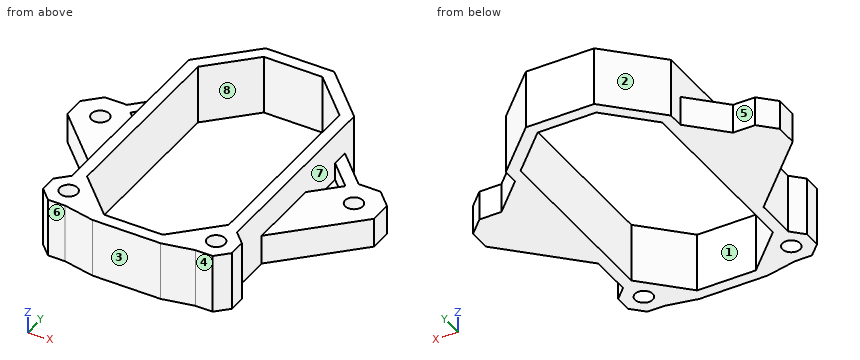
```python
from build123d import *

# Parameters (mm, degrees)
SKETCH2_R           = 1.5
BOSS_EXTRUDE1_DEPTH = 2
SKETCH5_R           = 1.5
BOSS_EXTRUDE4_DEPTH = 3
SKETCH6_R           = 1.5
BOSS_EXTRUDE5_DEPTH = 5


with BuildPart() as part:
    # Sketch2 → Boss-Extrude1 (new body)
    with BuildSketch(Plane.XY):
        Polygon((-26, -1.863961031), (-23.363961031, -4.5), (-14, -13.863961031), (-14, -20.798989873), (-14, -20.970562748), (-16, -22.970562748), (-16, -25.870057685), (-13.949747468, -27.920310217), (-11.050252532, -27.920310217), (-5.798989873, -29), (5.798989873, -29), (11.050252532, -27.920310217), (13.949747468, -27.920310217), (16, -25.870057685), (16, -22.970562748), (14, -20.970562748), (14, -20.798989873), (14, -13.863961031), (23.363961031, -4.5), (26, -1.863961031), (26, 1.863961031), (23.363961031, 4.5), (19.636038969, 4.5), (14, 10.136038969), (14, 12.798989873), (5.798989873, 21), (-5.798989873, 21), (-14, 12.798989873), (-14, 10.136038969), (-19.636038969, 4.5), (-23.363961031, 4.5), (-26, 1.863961031), align=None)
        with Locations((-12.5, -24.420310217)):
            Circle(SKETCH2_R, mode=Mode.SUBTRACT)
        with Locations(Location((12.5, -24.420310217, 0), (0, 0, 180))):
            Circle(SKETCH2_R, mode=Mode.SUBTRACT)
        Polygon((4.970562748, 19), (-4.970562748, 19), (-12, 11.970562748), (-12, 0), (-12, -19.970562748), (-4.970562748, -27), (4.970562748, -27), (12, -19.970562748), (12, 0), (12, 11.970562748), align=None, mode=Mode.SUBTRACT)
    extrude(amount=BOSS_EXTRUDE1_DEPTH)

    # Sketch5 → Boss-Extrude4 (add)
    with BuildSketch(Plane.XY.offset(2)):
        Polygon((-5.798989873, 21), (-14, 12.798989873), (-14, 10.136038969), (-19.636038969, 4.5), (-23.363961031, 4.5), (-26, 1.863961031), (-26, -1.863961031), (-23.363961031, -4.5), (-14, -13.863961031), (-14, -20.798989873), (-14, -20.970562748), (-16, -22.970562748), (-16, -25.870057685), (-13.949747468, -27.920310217), (-11.050252532, -27.920310217), (-5.798989873, -29), (5.798989873, -29), (11.050252532, -27.920310217), (13.949747468, -27.920310217), (16, -25.870057685), (16, -22.970562748), (14, -20.970562748), (14, -20.798989873), (14, -13.863961031), (23.363961031, -4.5), (26, -1.863961031), (26, 1.863961031), (23.363961031, 4.5), (19.636038969, 4.5), (14, 10.136038969), (14, 12.798989873), (5.798989873, 21), align=None)
        with Locations((-21.5, 0)):
            Circle(SKETCH5_R, mode=Mode.SUBTRACT)
        with Locations(Location((21.5, 0, 0), (0, 0, 180))):
            Circle(SKETCH5_R, mode=Mode.SUBTRACT)
        with Locations((-12.5, -24.420310217)):
            Circle(SKETCH5_R, mode=Mode.SUBTRACT)
        with Locations(Location((12.5, -24.420310217, 0), (0, 0, 180))):
            Circle(SKETCH5_R, mode=Mode.SUBTRACT)
        Polygon((-18.221825407, 3.085786438), (-14, 7.307611845), (-14, 0), (-14, -1.136038969), (-17, 1.863961031), align=None, mode=Mode.SUBTRACT)
        Polygon((4.970562748, -27), (-4.970562748, -27), (-12, -19.970562748), (-12, 0), (-12, 11.970562748), (-4.970562748, 19), (4.970562748, 19), (12, 11.970562748), (12, 0), (12, -19.970562748), align=None, mode=Mode.SUBTRACT)
        Polygon((14, -1.136038969), (14, 0), (14, 7.307611845), (18.221825407, 3.085786438), (17, 1.863961031), align=None, mode=Mode.SUBTRACT)
    extrude(amount=BOSS_EXTRUDE4_DEPTH)

    # Sketch6 → Boss-Extrude5 (add)
    with BuildSketch(Plane.XY.offset(5)):
        Polygon((5.798989873, -29), (-5.798989873, -29), (-11.050252532, -27.920310217), (-13.949747468, -27.920310217), (-16, -25.870057685), (-16, -22.970562748), (-14, -20.970562748), (-14, -20.798989873), (-14, 0), (-14, 12.798989873), (-5.798989873, 21), (5.798989873, 21), (14, 12.798989873), (14, 0), (14, -20.798989873), (14, -20.970562748), (16, -22.970562748), (16, -25.870057685), (13.949747468, -27.920310217), (11.050252532, -27.920310217), align=None)
        with Locations((-12.5, -24.420310217)):
            Circle(SKETCH6_R, mode=Mode.SUBTRACT)
        with Locations(Location((12.5, -24.420310217, 0), (0, 0, 180))):
            Circle(SKETCH6_R, mode=Mode.SUBTRACT)
        Polygon((4.970562748, 19), (-4.970562748, 19), (-12, 11.970562748), (-12, 0), (-12, -19.970562748), (-4.970562748, -27), (4.970562748, -27), (12, -19.970562748), (12, 0), (12, 11.970562748), align=None, mode=Mode.SUBTRACT)
    extrude(amount=BOSS_EXTRUDE5_DEPTH)


solid = part.part
```
The listing builds one solid part. Answer for the finished solid, in the listing's coordinates (mm). Face numbers are marked on the shaded views. A direction names the side the tool comes from. Coordinates: 2 decimals unless noted, no trailing zeros. Loops run counter-clockwise (first coordinate to the right, second up) from the corner with the lowest first, then second, coordinate; pieces in that order, holes last. Notation, with made-up numbers: (50.5, 48) -> (79.5, 48) arc R23 ccw to (79.5, 65) -> close; hole circle Ø3 at (28, 55.25). An arc over 180 degrees is marked (long way). Use one line per item in the form item = value. Start each with the question number.
Item 1: The part is cut by section A-A on x = 1. Determine the outline of the cut face in (y, z), then the cut area to 3 significant figures.
Item 2: Flat-ended cylindrical pins translate along their axes: pin 1 Ø2.5 at (x, y) = (-21.5, -0.5) entering from +Z; pin 2 Ø6 at (y, z) = (16, 8.5) entering from +X; pin 3 Ø2.5 at (y, z) = (-24.5, 6.5) entering from -X. Find the tip coordinate at first contact, or state that the pin passes through.
Item 3: The part is cut by section B-B on y = 13.5. Determine the outline of the cut face in (x, z).
Item 4: The mould has two halves that part along X. Classify the marked faces 1, 2 and 3: released by +X, released by -X, zero draft, split by the parting line, or undercut.
Item 5: The part is cut by section C-C on z = 6.5. Determine the outline of the cut face in (x, y).
Item 6: The part is cut by section D-D on y = -3.5. Determine the outline of the cut face in (x, z).
Item 7: Consider L1, parallel to X at y = 6.5, z = 6.25; L2, parallel to Y at x = 4, z = 3.5; L3, parallel to X at y = 17, z = 8. Determine where each line is inside the solid, lowest interval first. Write a range as [from, to].
Item 8: A tool of negligible diameter and unlimited length cuts with its end or side. For the marked faces 4, 5, 6, 7 and 8, from which of +Z, -Z, +X, -X, +Y, -Y can it reach the whole face along a straight path? Write none if from no direction.
Answer key:
q1.outline = (-29, 0) -> (-27, 0) -> (-27, 10) -> (-29, 10) -> close; (19, 0) -> (21, 0) -> (21, 10) -> (19, 10) -> close
q1.area = 40.0 mm2
q2.pin_1 = 5
q2.pin_2 = 13.8
q2.pin_3 = -16
q3.outline = (-13.3, 0) -> (-10.47, 0) -> (-10.47, 10) -> (-13.3, 10) -> close; (10.47, 0) -> (13.3, 0) -> (13.3, 10) -> (10.47, 10) -> close
q4.face_1 = undercut
q4.face_2 = released by -X
q4.face_3 = zero draft
q5.outline = (-16, -25.87) -> (-13.95, -27.92) -> (-11.05, -27.92) -> (-5.8, -29) -> (5.8, -29) -> (11.05, -27.92) -> (13.95, -27.92) -> (16, -25.87) -> (16, -22.97) -> (14, -20.97) -> (14, 12.8) -> (5.8, 21) -> (-5.8, 21) -> (-14, 12.8) -> (-14, -20.97) -> (-16, -22.97) -> close; hole circle Ø3 at (-12.5, -24.42); hole (-12, -19.97) -> (-4.97, -27) -> (4.97, -27) -> (12, -19.97) -> (12, 11.97) -> (4.97, 19) -> (-4.97, 19) -> (-12, 11.97) -> close; hole circle Ø3 at (12.5, -24.42)
q6.outline = (-24.36, 0) -> (-12, 0) -> (-12, 10) -> (-14, 10) -> (-14, 5) -> (-24.36, 5) -> close; (12, 0) -> (24.36, 0) -> (24.36, 5) -> (14, 5) -> (14, 10) -> (12, 10) -> close
q7.L1 = [-14, -12], [12, 14]
q7.L2 = [-29, -27], [19, 21]
q7.L3 = [-9.8, -6.97], [6.97, 9.8]
q8.face_4 = +Z, -Z, +X, -Y
q8.face_5 = +Z, -Z, -X, +Y
q8.face_6 = +Z, -Z, -X, -Y
q8.face_7 = +Z
q8.face_8 = +Z, -Z
